Input: part model. Units: mm. Frame: model coordinates. Face numbers are marked on the shaded views. A direction names the side the tool comes from. Round coordinates to 2 decimals unless told otherwise and drop trailing zeros. Loops run counter-clockwise (first coordinate to the right, second up) from the corner with the lowest first, then second, coordinate; pieces in that order, holes last. Notation, with made-up numbers: (24.5, 45) -> (64.5, 45) arc R23 cw to (64.5, 82) -> close; hole circle Ø4 at (76.5, 17.25). An arc over 180 degrees is marked (long way). Answer in a Markdown table with one row per item. Add a question column.
Q1. Section B-B, the plane z = 27.5. Output: boundary loops of the cut face in (x, y), and give its area (3 significant figures).
Q2. Section C-C, the plane y = 7.5. Output: boundary loops of the cut face in (x, z), and give its area (3 significant figures).
Q3. Reachability of the marked faces 1 and 2 from +Z, -Z, +X, -X, +Y, -Y: full face, straight path, thin tool, end or side. Return the list, or none.
Q4. Ray query, L1, parallel to Y at x = 6, z = 55; L2, parallel to Z at x = 19, y = 7; L3, parallel to Z at x = 2, y = 5.25. Return the intervals inside material, ascending. Write a range as from..to.
Q5. Pin query (flat end, axial travel): pin 1 (7.5 mm diameter, centred on x = 4.5, z = 21.5, fed in from +Y); pin 2 (3 mm diameter, centred on x = 7.6, z = 27.5, fed in from -Y); pin 3 (1.2 mm diameter, centred on y = -1.5, z = 21, fed in from -X); pin 4 (8 mm diameter, centred on x = 16, y = 12, fed in from +Z). Return the tip coordinate at first contact, or that it passes through.
Q6. Section D-D, the plane z = 12.5. Output: boundary loops of the cut face in (x, y), and give its area (3 significant figures).
Q7. Section A-A, the plane x = 7.6. Output: boundary loops of the cut face in (y, z), and give its area (3 significant figures).
```python
from build123d import *

# Parameters (mm, degrees)
BOSS_EXTRUDE1_DEPTH = 50
SKETCH2_W           = 25.4
SKETCH2_H           = 19
BOSS_EXTRUDE2_DEPTH = 25.4
SKETCH3_R           = 3.3
CUT_EXTRUDE1_DEPTH  = 25.4
SKETCH4_R           = 1.6
SKETCH4_R_2         = 1.60271378
CUT_EXTRUDE2_DEPTH  = 25.4
SKETCH5_R           = 1.746858549
SKETCH5_R_2         = 1.6
CUT_EXTRUDE3_DEPTH  = 20
SKETCH6_W           = 5.1
SKETCH6_H           = 47
CUT_EXTRUDE4_DEPTH  = 20
SKETCH7_W           = 15.2
SKETCH7_H           = 3
BOSS_EXTRUDE3_DEPTH = 15


with BuildPart() as part:
    # Sketch1 → Boss-Extrude1 (new body)
    with BuildSketch(Plane.XY):
        Polygon((0, 0), (0, 15), (-5.1, 15), (-5.1, -4), (20.3, -4), (20.3, 15), (15.2, 15), (15.2, 0), align=None)
    extrude(amount=BOSS_EXTRUDE1_DEPTH)

    # Sketch2 → Boss-Extrude2 (add)
    with BuildSketch(Plane.XY.offset(50)):
        with Locations((7.6, 5.5)):
            Rectangle(SKETCH2_W, SKETCH2_H)
    extrude(amount=BOSS_EXTRUDE2_DEPTH)

    # Sketch3 → Cut-Extrude1 (cut)
    with BuildSketch(Plane(origin=(20.3, 0, 0), x_dir=(0, 0, -1), z_dir=(1, 0, 0))):
        with Locations((-55, 5.5)):
            Circle(SKETCH3_R)
        with BuildLine():
            Line((-55, -4), (-75.4, -4))
            Line((-75.4, -4), (-75.4, 15))
            Line((-75.4, 15), (-55, 15))
            ThreePointArc((-55, 15), (-64.5, 5.5), (-55, -4))
        make_face()
    extrude(amount=-CUT_EXTRUDE1_DEPTH, mode=Mode.SUBTRACT)

    # Sketch4 → Cut-Extrude2 (cut)
    with BuildSketch(Plane(origin=(20.3, 0, 0), x_dir=(0, 0, -1), z_dir=(1, 0, 0))):
        with Locations((-12.5, 7.5)):
            Circle(SKETCH4_R)
        with Locations((-27.5, 7.5)):
            Circle(SKETCH4_R_2)
    extrude(amount=-CUT_EXTRUDE2_DEPTH, mode=Mode.SUBTRACT)

    # Sketch5 → Cut-Extrude3 (cut, through all)
    with BuildSketch(Plane.XZ.offset(4)):
        with Locations((7.6, 12.5)):
            Circle(SKETCH5_R)
        with Locations((7.6, 27.5)):
            Circle(SKETCH5_R_2)
    extrude(amount=-CUT_EXTRUDE3_DEPTH, mode=Mode.SUBTRACT)

    # Sketch6 → Cut-Extrude4 (cut, through all)
    with BuildSketch(Plane(origin=(0, 15, 0), x_dir=(1, 0, 0), z_dir=(0, 1, 0))):
        with Locations((-2.55, -23.5)):
            Rectangle(SKETCH6_W, SKETCH6_H)
    extrude(amount=-CUT_EXTRUDE4_DEPTH, mode=Mode.SUBTRACT)

    # Sketch7 → Boss-Extrude3 (add)
    with BuildSketch(Plane(origin=(0, 0, 0), x_dir=(1, 0, 0), z_dir=(0, 1, 0))):
        with Locations((7.6, -48.5)):
            Rectangle(SKETCH7_W, SKETCH7_H)
    extrude(amount=BOSS_EXTRUDE3_DEPTH)


solid = part.part
```
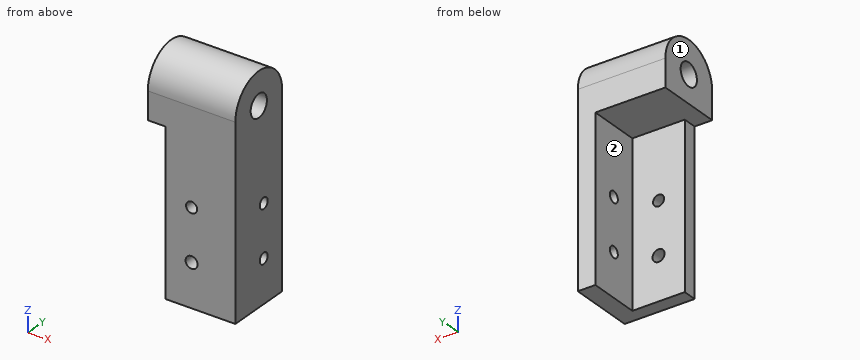
Answer block:
| question | item | result |
|---|---|---|
| 1 | outline | (0, -4) -> (6, -4) -> (6, 0) -> (0, 0) -> close; (9.2, -4) -> (20.3, -4) -> (20.3, 5.9) -> (15.2, 5.9) -> (15.2, 0) -> (9.2, 0) -> close; (15.2, 9.1) -> (20.3, 9.1) -> (20.3, 15) -> (15.2, 15) -> close |
| 1 | area | 129 mm^2 |
| 2 | outline | (-5.1, 47) -> (15.2, 47) -> (15.2, 29.1) -> (20.3, 29.1) -> (20.3, 52.38) -> (-5.1, 52.38) -> close; (-5.1, 57.62) -> (20.3, 57.62) -> (20.3, 64.29) -> (-5.1, 64.29) -> close; (15.2, 0) -> (20.3, 0) -> (20.3, 10.9) -> (15.2, 10.9) -> close; (15.2, 14.1) -> (20.3, 14.1) -> (20.3, 25.9) -> (15.2, 25.9) -> close |
| 2 | area | 513 mm^2 |
| 3 | face 1 | +Z, -Z, -X, +Y, -Y |
| 3 | face 2 | -Z, -X, +Y |
| 4 | L1 | -4..2.2, 8.8..15 |
| 4 | L2 | 0..10.98, 14.02..25.98, 29.02..52.06, 57.94..64.38 |
| 4 | L3 | 47..51.71, 58.29..64.5 |
| 5 | pin 1 | y = 0 |
| 5 | pin 2 | through |
| 5 | pin 3 | x = 0 |
| 5 | pin 4 | z = 64.17 |
| 6 | outline | (0, -4) -> (5.85, -4) -> (5.85, 0) -> (0, 0) -> close; (9.35, -4) -> (20.3, -4) -> (20.3, 5.9) -> (15.2, 5.9) -> (15.2, 0) -> (9.35, 0) -> close; (15.2, 9.1) -> (20.3, 9.1) -> (20.3, 15) -> (15.2, 15) -> close |
| 6 | area | 127 mm^2 |
| 7 | outline | (-4, 0) -> (0, 0) -> (0, 10.75) -> (-4, 10.75) -> close; (-4, 14.25) -> (0, 14.25) -> (0, 25.9) -> (-4, 25.9) -> close; (-4, 29.1) -> (0, 29.1) -> (0, 47) -> (15, 47) -> (15, 55) arc R9.5 ccw to (-4, 55) -> close; hole circle Ø6.6 at (5.5, 55) |
| 7 | area | 421 mm^2 |
